Verification items for the finished model (mm, model axes). Face numbers are marked on the shaded views. A direction names the side the tool comes from. Round coordinates to 2 decimals unless told otherwise and drop trailing zeros. Write each loop counter-clockwise with the first axis right and the second up, starting at its lowest first coordinate (ties: lowest second). Pieces come first, ordered by that corner, then holes. Notation, with made-up numbers: M -31.75,28.25 L 13.25,28.25 A19 cw 13.25,37.25 Z; hole C 33,5.25 d9. An arc over 180 degrees is marked long. One line per question, with ' | ' between items. Start each with the question number.
Q1. Thickness scan on line 1 along X through (y, z) = (2.15, 0); line 2 along X through (y, z) = (0.5, 0.5). Record the ranges inside material, lowest first. Write a range as from..to.
Q2. Release check for a two-part mould opening along Z. For the marked faces 1, 2 and 3 record: released by +Z, released by -Z, zero draft, split by the parting line, or undercut.
Q3. Cross-section at C-C (y = 2.65). Record the boundary of the cut face in (x, z), then the cut area to 3 significant figures.
Q4. Cross-section at D-D (y = 0.7). Record the boundary of the cut face in (x, z), then the cut area to 3 significant figures.
Q5. Gauge pin test, flat ends, axial feed: pin 1 (1 mm diameter, centred on y = 1, z = 1, fed in from +X); pin 2 (3.5 mm diameter, centred on x = 0.5, z = 0, fed in from +Y). Record the tip position at first contact, or that the pin passes through.
Q6. Cross-section at A-A (z = 0). Record the boundary of the cut face in (x, y).
Q7. Tool access check on the marked faces 4 and 5. Record the directions out of +Z, -Z, +X, -X, +Y, -Y that give a thin tool (end or side, any length) a straight path to the whole face; none if there is none.
Q8. Cross-section at B-B (x = 0). Record the boundary of the cut face in (y, z).
Autodesk Inventor part; units mm, degrees
ref_plane "YZ Plane" through (0, 0, 0) normal (1, 0, 0) x (0, 1, 0)
ref_plane "XZ Plane" through (0, 0, 0) normal (0, 1, 0) x (-1, 0, 0)
ref_plane "XY Plane" through (0, 0, 0) normal (0, 0, 1) x (1, 0, 0)
sketch "Sketch1" plane through (0, 0, 0) normal (0, 1, 0) x (-1, 0, 0)
  circle A0 centre (0, 0) radius 3.3
  dimension "d0" = 6.6
extrude "Extrusion1" add sketch "Sketch1" along normal blind 1
sketch "Sketch2" plane through (0, 1, 0) normal (0, 1, 0) x (1, 0, 0)
  point P0 (0, 0)
sketch "Sketch3" plane through (0, 1, 0) normal (0, 1, 0) x (1, 0, 0)
  circle A0 centre (0, 0) radius 2.5
  dimension "d3" = 5
extrude "Extrusion2" add sketch "Sketch3" along normal blind 2
sketch "Sketch4" plane through (0, 3, 0) normal (0, 1, 0) x (1, 0, 0)
  circle A0 centre (0, 0) radius 1.5
  dimension "d6" = 3
extrude "Extrusion3" cut sketch "Sketch4" against normal blind 3
thread "Thread1"
properties part number "HAND_persely"
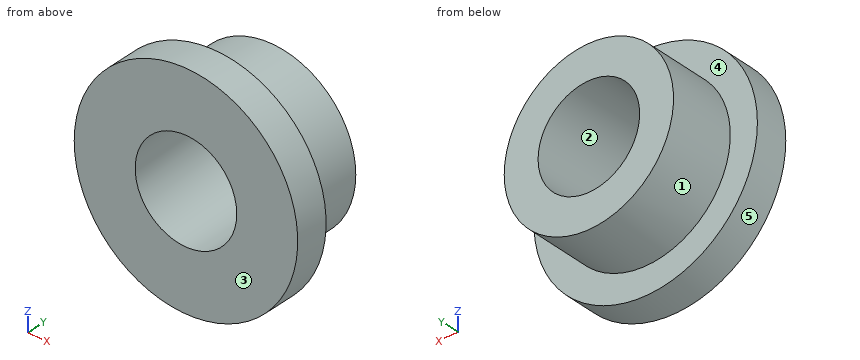
Determined:
1) line 1: x = -2.5..-1.5, 1.5..2.5 | line 2: x = -3.26..-1.41, 1.41..3.26
2) face 1: split by the parting line | face 2: undercut | face 3: zero draft
3) outline: C 0,0 d5; hole C 0,0 d3 | area: 12.6 mm²
4) outline: C 0,0 d6.6; hole C 0,0 d3 | area: 27.1 mm²
5) pin 1: stops at x = 3.26 | pin 2: stops at y = 3
6) outline: M -3.3,0 L -1.5,0 L -1.5,3 L -2.5,3 L -2.5,1 L -3.3,1 Z; M 1.5,0 L 3.3,0 L 3.3,1 L 2.5,1 L 2.5,3 L 1.5,3 Z
7) face 4: +Y | face 5: +Y, -Y
8) outline: M 0,-3.3 L 1,-3.3 L 1,-2.5 L 3,-2.5 L 3,-1.5 L 0,-1.5 Z; M 0,1.5 L 3,1.5 L 3,2.5 L 1,2.5 L 1,3.3 L 0,3.3 Z
